Geometry check sheet. Reference: the model listing, model coordinates, mm. Face numbers are marked on the shaded views. A direction names the side the tool comes from. Give positions to 0.01 mm unless a question says otherwise; leave off trailing zeros. Loops run counter-clockwise (first coordinate to the right, second up) from the corner with the lowest first, then second, coordinate; pieces in that order, holes last. Notation, with made-up numbers: (15, -27) - (43, -27) arc R30 cw to (43, -4) - close; hole circle Ø4 at (-31.5, -19.75). An arc over 180 degrees is marked (long way). Use a Markdown table: item, result. Add a question column.
1. Material ranges on L1, parallel to Z at x = -12.25, y = 0; L2, parallel to Y at x = -11, z = 4; L3, parallel to Z at x = -25.75, y = 1, recorded low to high.
2. Set-up check for the marked faces 4 and 5: record each of +Z, -Z, +X, -X, +Y, -Y from which the full face is reachable in a straight line by a thin tool's end or side.
3. Cross-section at A-A on x = -3.25. Enter the section's corners in (y, z), and give its area (3 significant figures).
4. Draft check along Z on the marked faces 1, 2 and 3. Enter one of: pulls with the +Z half, pulls with the -Z half, needs draft (parallel to the pull), parting line crosses it, or undercut.
5. Cross-section at B-B on x = -26.5. Enter the section's corners in (y, z), and give its area (3 significant figures).
6. Depth check by flat-ended pin: P1, Ø5, axis at x = -5.5, y = 3, coming from the -Z side; P2, Ø10, axis at x = -16.5, z = -11.5, coming from the +Y side; P3, Ø10, axis at x = -6.5, z = -12, coming from the +Y side. Enter the tip coordinate at first touch or a pass-through.
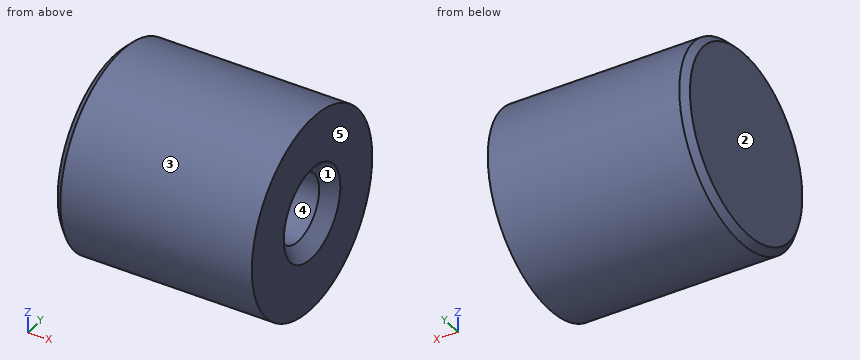
Autodesk Inventor part; units mm, degrees
ref_plane "YZ Plane" through (0, 0, 0) normal (1, 0, 0) x (0, 1, 0)
ref_plane "XZ Plane" through (0, 0, 0) normal (0, 1, 0) x (-1, 0, 0)
ref_plane "XY Plane" through (0, 0, 0) normal (0, 0, 1) x (1, 0, 0)
sketch "Sketch1" plane through (0, 0, 0) normal (0, 0, 1) x (1, 0, 0)
  line L0 (-36, 0) -> (6, 0)
  line L1 (0, -3) -> (0, 18) construction
  line L2 (0, 0) -> (0, 15)
  line L3 (0, 15) -> (-30, 15)
  line L4 (-30, 15) -> (-30, 0)
  dimension "d0" = 30
  dimension "d1" = 30
revolve "Revolution1" add sketch "Sketch1" angle 360 about axis through (-10, 0, 0) along (1, 0, 0)
sketch "Sketch2" plane through (0, 0, 0) normal (1, 0, 0) x (0, 0, -1)
  circle A0 centre (0, 0) radius 15
hole "Hole1" at (0, 0, 0) direction (-1, 0, 0) diameter 10.106 depth 15 tip angle 118 countersink diameter 14.1 countersink angle 90
chamfer "Chamfer1" distance 1 angle 45 1 edges at (-30, -15, 0)
properties part number "HM1-003X"
Values found:
| question | item | result |
|---|---|---|
| 1 | L1 | z = -15 to -5.05, 5.05 to 15 |
| 1 | L2 | y = -14.46 to -3.09, 3.09 to 14.46 |
| 1 | L3 | z = -14.97 to 14.97 |
| 2 | face 4 | +X |
| 2 | face 5 | +Z, -Z, +X, +Y, -Y |
| 3 | outline | circle Ø30 at (0, 0); hole circle Ø10.11 at (0, 0) |
| 3 | area | 627 mm2 |
| 4 | face 1 | undercut |
| 4 | face 2 | needs draft |
| 4 | face 3 | parting line crosses it |
| 5 | outline | circle Ø30 at (0, 0) |
| 5 | area | 707 mm2 |
| 6 | P1 | stops at z = -14.99 |
| 6 | P2 | stops at y = 13.52 |
| 6 | P3 | stops at y = 13.27 |
